For this review, take the finished solid that the model builds, in its own axes (mm). Face numbers are marked on the shaded views. A direction names the side the tool comes from. Round coordinates to 2 decimals unless told otherwise and drop trailing zeros. Order: outer loops, then holes, each group sorted by start corner. A loop starts at its lowest first (then second) coordinate and runs counter-clockwise, first axis right, second up. Notation, with made-up numbers: M 54,7 L 91,7 A15 cw 91,12 Z; hole C 12,-39 d6. An arc over 180 degrees is marked long. Answer in a Markdown table with one row per item. Add a question column.
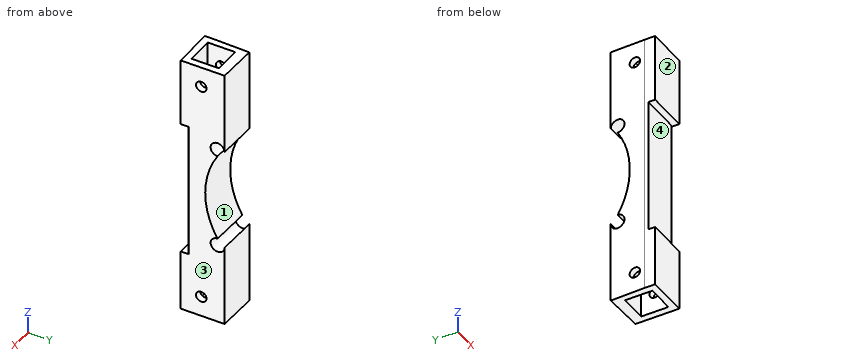
```python
from build123d import *

# Parameters (mm, degrees)
PAD_DEPTH       = 80
POCKET_DEPTH    = 78
POCKET001_DEPTH = 408.7079232475
POCKET002_DEPTH = 408.4326470939
SKETCH004_W     = 433.609177
SKETCH004_H     = 149.2376851805
SKETCH004_W_2   = 114.034424
SKETCH004_H_2   = 150.6867891805
POCKET003_DEPTH = 80.001
SKETCH005_W     = 8
SKETCH005_H     = 8
POCKET004_DEPTH = 10
SKETCH006_W     = 8
SKETCH006_H     = 8
POCKET005_DEPTH = 12
SKETCH007_R     = 1.55
POCKET006_DEPTH = 12.001
POCKET007_DEPTH = 12.001
SKETCH009_W     = 2
SKETCH009_H     = 40
POCKET008_DEPTH = 12.001
FILLET_R        = 0.5


with BuildPart() as part:
    # Sketch → Pad (new body)
    with BuildSketch(Plane.XY):
        Polygon((450, 0), (450, 90), (356, 87.18), (355.64, 99.18), (343.64, 98.82), (344, 86.82), (6, 76.68), (5.64, 88.6800000001), (-6.36, 88.3200000001), (-6, 76.32), (-50, 75), (-50, 0), align=None)
    extrude(amount=PAD_DEPTH)

    # Sketch001 (on Face14 of Pad) → Pocket (cut)
    with BuildSketch(Plane.XY.offset(80)):
        Polygon((-50, 15), (-50, 74), (450, 74), (450, 0), (356, 2.82), (356.3, 12.82), (344.3, 13.18), (344, 3.18), (6, 13.32), (6.3, 23.32), (-5.7, 23.68), (-6, 13.68), align=None)
    extrude(amount=-POCKET_DEPTH, mode=Mode.SUBTRACT)

    # Sketch002 (on Face26 of Pocket) → Pocket001 (cut, through all)
    with BuildSketch(Plane(origin=(355.5953641722, -10.6678609252, 0), x_dir=(0.0299865091, 0.9995503035, 0), z_dir=(0.9995503035, -0.0299865091, 0))):
        with BuildLine():
            ThreePointArc((23.4984280855, 56), (19.9988591841, 57.4495689014), (21.4484280855, 53.95))
            ThreePointArc((21.4484280855, 53.95), (17.8329435114, 41), (21.4484280855, 28.05))
            ThreePointArc((21.4484280855, 28.05), (19.9988591841, 24.5504310986), (23.4984280855, 26))
            Line((23.4984280855, 26), (23.4984280855, 56))
        make_face()
    extrude(amount=-POCKET001_DEPTH, mode=Mode.SUBTRACT)

    # Sketch003 (on Face14 of Pocket001) → Pocket002 (cut, through all)
    with BuildSketch(Plane(origin=(358.2929363573, 10.7487880907, 0), x_dir=(-0.0299865091, 0.9995503035, 0), z_dir=(0.9995503035, 0.0299865091, 0))):
        with BuildLine():
            ThreePointArc((88.470997005, 56), (84.9714281036, 57.4495689014), (86.420997005, 53.95))
            ThreePointArc((86.420997005, 53.95), (82.8055124309, 41), (86.420997005, 28.05))
            ThreePointArc((86.420997005, 28.05), (84.9714281036, 24.5504310986), (88.470997005, 26))
            Line((88.470997005, 26), (88.470997005, 56))
        make_face()
    extrude(amount=-POCKET002_DEPTH, mode=Mode.SUBTRACT)

    # Sketch004 (on Face7 of Pocket002) → Pocket003 (cut, through all)
    with BuildSketch(Plane.XY.offset(80)):
        with Locations((127.1954115, 57.2464115903)):
            Rectangle(SKETCH004_W, SKETCH004_H)
        with Locations((413.017212, 56.5218595903)):
            Rectangle(SKETCH004_W_2, SKETCH004_H_2)
    extrude(amount=-POCKET003_DEPTH, mode=Mode.SUBTRACT)

    # Sketch005 (on Face8 of Pocket003) → Pocket004 (cut)
    with BuildSketch(Plane.XY.offset(80)):
        with Locations((350, 88)):
            Rectangle(SKETCH005_W, SKETCH005_H)
        with Locations((350, 6)):
            Rectangle(SKETCH005_W, SKETCH005_H)
    extrude(amount=-POCKET004_DEPTH, mode=Mode.SUBTRACT)

    # Sketch006 (on Face1 of Pocket004) → Pocket005 (cut)
    with BuildSketch(Plane(origin=(0, 0, 0), x_dir=(1, 0, 0), z_dir=(0, 0, -1))):
        with Locations((350, -6)):
            Rectangle(SKETCH006_W, SKETCH006_H)
        with Locations((350, -88)):
            Rectangle(SKETCH006_W, SKETCH006_H)
    extrude(amount=-POCKET005_DEPTH, mode=Mode.SUBTRACT)

    # Sketch007 (on Face6 of Pocket005) → Pocket006 (cut, through all)
    with BuildSketch(Plane.YZ.offset(356)):
        with Locations((6, 74)):
            Circle(SKETCH007_R)
        with Locations((88, 74)):
            Circle(SKETCH007_R)
        with Locations((88, 8)):
            Circle(SKETCH007_R)
        with Locations((6, 8)):
            Circle(SKETCH007_R)
    extrude(amount=-POCKET006_DEPTH, mode=Mode.SUBTRACT)

    # Sketch008 (on Face2 of Pocket006) → Pocket007 (cut, through all)
    with BuildSketch(Plane(origin=(344, 0, 0), x_dir=(0, -1, 0), z_dir=(-1, 0, 0))):
        Polygon((-136.047638, 92.811623), (-13.18, 92.811623), (-13.18, 2), (21.701658, 2), (21.701658, -28.608723), (-136.047638, -28.608723), align=None)
    extrude(amount=-POCKET007_DEPTH, mode=Mode.SUBTRACT)

    # Sketch009 (on Face13 of Pocket007) → Pocket008 (cut, through all)
    with BuildSketch(Plane.YZ.offset(356)):
        with Locations((1, 40)):
            Rectangle(SKETCH009_W, SKETCH009_H)
    extrude(amount=-POCKET008_DEPTH, mode=Mode.SUBTRACT)

    # Fillet
    fillet_edges = [part.edges().sort_by_distance(p)[0] for p in [
        (356, 2, 40),
    ]]
    fillet(fillet_edges, radius=FILLET_R)


solid = part.part
```
1. Clearance check with flat-ended pins moving along their axes: pin 1 Ø1.9 at (y, z) = (6, 8) entering from -X; pin 2 Ø6.5 at (x, z) = (350.5, 5) entering from +Y; pin 3 Ø6 at (x, y) = (352, 5) entering from -Z; pin 4 Ø3.5 at (x, z) = (352.5, 46.5) entering from -Y. State where each tip first meets the part, or that it passes through.
2. Consider section A-A on z = 8. Write out the cut boundary in (x, y).
3. Consider section D-D on z = 55. Write out the cut boundary in (x, y), plus the area to 3 significant figures.
4. Consider section C-C on z = 64.5. Write out the cut boundary in (x, y).
5. The part is to be moulded in two halves that separate along Z. For the marked faces 1 and 2, say which applies: pulls with the +Z half, pulls with the -Z half, needs draft (parallel to the pull), parting line crosses it, or undercut.
6. For the marked faces 3 and 4, list the 3-axis set-ups (+Z, -Z, +X, -X, +Y, -Y) from which the entire face can be reached by the end or side of a thin tool; tool diameter is ignored.
7. Consider section B-B on y = 6. Write out the cut boundary in (x, z), plus the area to 3 significant figures.
8. To check wall thickness, follow probe 1 along Z at (x, y) = (354.7, 6); probe 2 along Z at (x, y) = (351, 10.5); probe 3 along Z at (x, y) = (355.25, 10.25). State the ranges of each line that lie inside material, in increasing order. Write a range as [from, to].
Solved:
| question | item | result |
|---|---|---|
| 1 | pin 1 | passes through |
| 1 | pin 2 | stops at y = 13.09 |
| 1 | pin 3 | stops at z = 2 |
| 1 | pin 4 | stops at y = 2 |
| 2 | outline | M 344,0 L 356,0 L 356,4.45 L 354,4.45 L 354,2 L 346,2 L 346,4.45 L 344.04,4.45 L 344,3.18 Z; M 344.13,7.55 L 346,7.55 L 346,10 L 354,10 L 354,7.55 L 356,7.55 L 356,12.83 L 344.3,13.18 Z |
| 3 | outline | M 344,2 L 355.5,2 A0.5 ccw 356,2.5 L 356,8.99 L 344.18,9.34 L 344,3.18 Z |
| 3 | area | 85.4 mm^2 |
| 4 | outline | M 344,0 L 356,0 L 356,12.83 L 344.3,13.18 L 344,3.18 Z |
| 5 | face 1 | undercut |
| 5 | face 2 | needs draft |
| 6 | face 3 | +Z, -Z, +X, +Y, -Y |
| 6 | face 4 | +X, -X, -Y |
| 7 | outline | M 344.08,2 L 346,2 L 346,6.45 L 344.08,6.45 Z; M 344.08,9.55 L 346,9.55 L 346,12 L 354,12 L 354,9.55 L 356,9.55 L 356,72.45 L 354,72.45 L 354,70 L 346,70 L 346,72.45 L 344.08,72.45 Z; M 344.08,75.55 L 346,75.55 L 346,80 L 344.08,80 Z; M 354,2 L 356,2 L 356,6.45 L 354,6.45 Z; M 354,75.55 L 356,75.55 L 356,80 L 354,80 Z |
| 7 | area | 745 mm^2 |
| 8 | probe 1 | z = [2, 6.45], [9.55, 72.45], [75.55, 80] |
| 8 | probe 2 | z = [2, 24], [28, 28.78], [53.22, 54], [58, 80] |
| 8 | probe 3 | z = [2, 24.03], [27.97, 29.01], [52.99, 54.03], [57.97, 80] |
